Input: part model. Units: mm. Frame: model coordinates. Face numbers are marked on the shaded views. Give positions to 0.01 mm unless a question says otherwise; leave off trailing zeros. Order: outer loops, then holes, each group sorted by start corner. A loop starts at its lowest first (then second) coordinate and runs counter-clockwise, first axis right, second up. Notation, with made-up numbers: M 42.5,-32 L 82.5,-32 A6 cw 82.5,-26 Z; hole C 74.25,-25 d2. An arc over 180 degrees is marked long. Use a Markdown table: item, result.
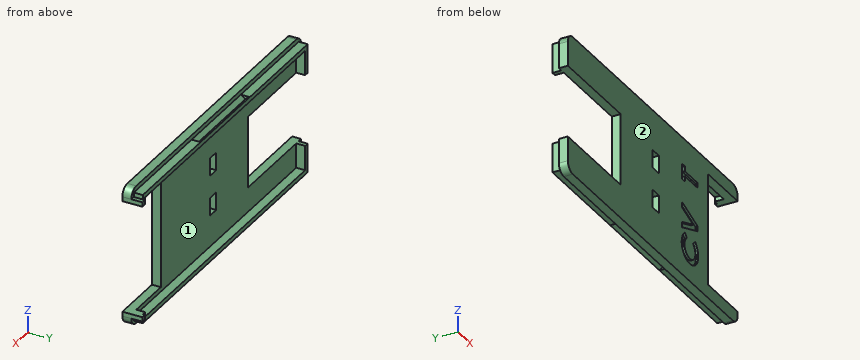
from build123d import *

# Parameters (mm, degrees)
BOSS_EXTRUDE1_DEPTH = 1
SKETCH3_W           = 67
SKETCH3_H           = 29
SKETCH3_W_2         = 65
SKETCH3_H_2         = 27
BOSS_EXTRUDE2_DEPTH = 2
CUT_EXTRUDE1_DEPTH  = 10
SKETCH7_W           = 21.5
SKETCH7_H           = 16
SKETCH7_W_2         = 12
SKETCH7_H_2         = 25
CUT_EXTRUDE2_DEPTH  = 20
SKETCH11_W          = 1
SKETCH11_H          = 1
BOSS_EXTRUDE5_DEPTH = 2.5
CUT_EXTRUDE3_DEPTH  = 0.5
SKETCH13_W          = 2.5
SKETCH13_H          = 4
CUT_EXTRUDE4_DEPTH  = 39.08871237


with BuildPart() as part:
    # Sketch1 → Boss-Extrude1 (new, symmetric)
    with BuildSketch(Plane(origin=(0, 0, 0), x_dir=(1, 0, 0), z_dir=(0, 1, 0))):
        with BuildLine():
            Line((-32.5, -15.5), (32.5, -15.5))
            ThreePointArc((32.5, -15.5), (33.914213562, -14.914213562), (34.5, -13.5))
            Line((34.5, -13.5), (34.5, 13.5))
            ThreePointArc((34.5, 13.5), (33.914213562, 14.914213562), (32.5, 15.5))
            Line((32.5, 15.5), (-32.5, 15.5))
            ThreePointArc((-32.5, 15.5), (-33.914213562, 14.914213562), (-34.5, 13.5))
            Line((-34.5, 13.5), (-34.5, -13.5))
            ThreePointArc((-34.5, -13.5), (-33.914213562, -14.914213562), (-32.5, -15.5))
        make_face()
    extrude(amount=BOSS_EXTRUDE1_DEPTH, both=True)

    # Sketch3 → Boss-Extrude2 (add)
    with BuildSketch(Plane(origin=(0, 1, 0), x_dir=(1, 0, 0), z_dir=(0, 1, 0))):
        Rectangle(SKETCH3_W, SKETCH3_H)
        Rectangle(SKETCH3_W_2, SKETCH3_H_2, mode=Mode.SUBTRACT)
    extrude(amount=BOSS_EXTRUDE2_DEPTH)

    # Sketch6 → Cut-Extrude1 (cut, symmetric)
    with BuildSketch(Plane(origin=(0, 0, 0), x_dir=(0, 0, -1), z_dir=(1, 0, 0))):
        Polygon((14.5, 1), (14.5, 3), (13.75, 2), align=None)
        Polygon((-13.75, 2), (-14.5, 1), (-14.5, 3), align=None)
    extrude(amount=CUT_EXTRUDE1_DEPTH, both=True, mode=Mode.SUBTRACT)

    # Sketch7 → Cut-Extrude2 (cut)
    with BuildSketch(Plane.XZ.offset(1)):
        with Locations((-23.75, 0)):
            Rectangle(SKETCH7_W, SKETCH7_H)
        with Locations((28.5, 0)):
            Rectangle(SKETCH7_W_2, SKETCH7_H_2)
    extrude(amount=-CUT_EXTRUDE2_DEPTH, mode=Mode.SUBTRACT)

    # Sketch11 → Boss-Extrude5 (add)
    with BuildSketch(Plane(origin=(0, 1, 0), x_dir=(1, 0, 0), z_dir=(0, 1, 0))):
        with Locations((34, 13)):
            Rectangle(SKETCH11_W, SKETCH11_H)
        with Locations((34, -13)):
            Rectangle(SKETCH11_W, SKETCH11_H)
    extrude(amount=BOSS_EXTRUDE5_DEPTH)

    # Sketch12 → Cut-Extrude3 (cut)
    with BuildSketch(Plane.XZ.offset(1)):
        Polygon((11.941533437, 6.065064103), (11.941533437, 9.484294872), (13.081277027, 9.484294872), (13.081277027, 8.344551282), (18.291533437, 8.344551282), (18.291533437, 7.204807692), (13.081277027, 7.204807692), (13.081277027, 6.065064103), align=None)
        Polygon((11.941533437, -4.884615385), (11.941533437, -3.667277644), (16.452170457, -2.03525641), (11.941533437, -0.399419071), (11.941533437, 0.814102564), (18.291533437, -1.48828125), (18.291533437, -2.586047676), align=None)
        with BuildLine():
            Line((13.043115969, -5.495192308), (13.84195411, -6.330919471))
            add(Edge.make_bspline(
                [(13.84195411, -6.330919471), (13.768637735, -6.401806055), (13.625427884, -6.540269761), (13.436040425, -6.763499644), (13.277548365, -6.995057512), (13.146745209, -7.232632751), (13.043791904, -7.47669033), (12.970992617, -7.72804876), (12.926114938, -7.986340764), (12.921019422, -8.161199427), (12.918456514, -8.249148638)],
                knots=[0, 0, 0, 0, 1.115315123, 2.178559852, 3.196385012, 4.180486591, 5.141138664, 6.08807191, 7.038351522, 8, 8, 8, 8], degree=3))
            add(Edge.make_bspline(
                [(12.918456514, -8.249148638), (12.920487286, -8.322594137), (12.92449479, -8.467530739), (12.953944547, -8.680315542), (13.00383624, -8.883932376), (13.07318533, -9.078542785), (13.160519089, -9.265108945), (13.270291327, -9.441893594), (13.398838264, -9.609846789), (13.545934957, -9.767006139), (13.707838119, -9.908887036), (13.878351171, -10.03672374), (14.060490077, -10.142609994), (14.251598692, -10.229044823), (14.451746028, -10.297157456), (14.660922066, -10.345499724), (14.879599088, -10.373509267), (15.028259493, -10.377685306), (15.103813085, -10.379807692)],
                knots=[0, 0, 0, 0, 1.035268443, 2.04298821, 3.02163646, 3.985902049, 4.951223231, 5.920091634, 6.913651787, 7.92868536, 8.949353712, 9.945284791, 10.92850487, 11.913014323, 12.897904816, 13.904240668, 14.934873455, 16, 16, 16, 16], degree=3))
            add(Edge.make_bspline(
                [(15.103813085, -10.379807692), (15.156840057, -10.379186533), (15.261357308, -10.377962216), (15.415574733, -10.364925614), (15.565507754, -10.343215337), (15.710796025, -10.312972773), (15.851629254, -10.274204313), (15.988337217, -10.229420059), (16.119289945, -10.172219135), (16.24693936, -10.109298874), (16.368212678, -10.036911087), (16.483189742, -9.95764624), (16.591896287, -9.872234836), (16.693945792, -9.779536195), (16.787869185, -9.678383039), (16.876223869, -9.571218373), (16.957616144, -9.456977598), (17.030749894, -9.335614926), (17.098918302, -9.210802926), (17.155368302, -9.07997032), (17.206114124, -8.94677674), (17.244290102, -8.808884538), (17.277495177, -8.66872294), (17.29777454, -8.524340956), (17.313184177, -8.377108845), (17.31413292, -8.277600269), (17.31461036, -8.227524038)],
                knots=[0, 0, 0, 0, 1.103738238, 2.175490744, 3.219137561, 4.256155604, 5.262629953, 6.259184223, 7.247888397, 8.234817694, 9.220364322, 10.185094651, 11.140491148, 12.096499151, 13.05201798, 14.011605636, 14.986460005, 15.968997565, 16.960259839, 17.944382265, 18.933125845, 19.924977513, 20.920749559, 21.929466621, 22.958034467, 24, 24, 24, 24], degree=3))
            add(Edge.make_bspline(
                [(17.31461036, -8.227524038), (17.312162797, -8.142583361), (17.307353971, -7.975697017), (17.269475061, -7.730825721), (17.207829637, -7.497111584), (17.132929858, -7.311049721), (17.060303901, -7.165191721), (16.995016409, -7.053220916), (16.919750327, -6.938662767), (16.834193119, -6.821691737), (16.738718629, -6.701628906), (16.631461316, -6.58046115), (16.51588805, -6.45512538), (16.43340391, -6.373017633), (16.391112764, -6.330919471)],
                knots=[0, 0, 0, 0, 1.404693586, 2.759857621, 4.088769373, 5.395275838, 6.0697462, 6.783214465, 7.53810233, 8.336454657, 9.18000028, 10.074808326, 11.012918585, 12, 12, 12, 12], degree=3))
            Line((16.391112764, -6.330919471), (17.242104351, -5.520633013))
            add(Edge.make_bspline(
                [(17.242104351, -5.520633013), (17.297096261, -5.577591789), (17.404428711, -5.68876314), (17.556830773, -5.856462037), (17.693780967, -6.023949878), (17.820249986, -6.187180506), (17.93255348, -6.348827808), (18.030803608, -6.508874644), (18.117485256, -6.665509211), (18.191136583, -6.821984078), (18.253674209, -6.979272912), (18.307515, -7.141104638), (18.353062372, -7.307973991), (18.38981312, -7.480900133), (18.419282258, -7.658270114), (18.439173756, -7.841743881), (18.452546148, -8.030158121), (18.453747768, -8.157962419), (18.45435395, -8.222435897)],
                knots=[0, 0, 0, 0, 1.244526981, 2.429050516, 3.560637417, 4.644440555, 5.67424972, 6.652764056, 7.595344123, 8.486817594, 9.369275933, 10.254498637, 11.166417451, 12.086725134, 13.032340136, 13.991389299, 14.986715468, 16, 16, 16, 16], degree=3))
            add(Edge.make_bspline(
                [(18.45435395, -8.222435897), (18.451334939, -8.340865691), (18.445427572, -8.572599876), (18.401657986, -8.912200283), (18.328279045, -9.234811554), (18.224500984, -9.541218541), (18.091929374, -9.831323814), (17.929402805, -10.105053156), (17.737353086, -10.361965375), (17.518031224, -10.599985126), (17.275808639, -10.815285319), (17.015728035, -11.005585757), (16.736511209, -11.163002287), (16.442283088, -11.293708623), (16.131700993, -11.395919259), (15.804428969, -11.467858219), (15.460783018, -11.51222245), (15.226064912, -11.51707596), (15.106357155, -11.519551282)],
                knots=[0, 0, 0, 0, 1.078019885, 2.10938526, 3.111377082, 4.085535484, 5.04941344, 6.010039228, 6.978205633, 7.964457913, 8.951525778, 9.924444315, 10.892603023, 11.863865945, 12.85144698, 13.863884204, 14.910567087, 16, 16, 16, 16], degree=3))
            add(Edge.make_bspline(
                [(15.106357155, -11.519551282), (15.028282903, -11.518515641), (14.873558818, -11.516463254), (14.645252317, -11.494488037), (14.422973185, -11.464639878), (14.208620877, -11.415608228), (13.999755502, -11.358606766), (13.798225395, -11.285168838), (13.603181636, -11.199848512), (13.414870564, -11.102428539), (13.235325687, -10.990848613), (13.063401988, -10.869367728), (12.901326556, -10.735039657), (12.748431173, -10.589223971), (12.602984036, -10.433268126), (12.468562175, -10.264501174), (12.341559366, -10.085801372), (12.225763331, -9.895930835), (12.120448829, -9.699216136), (12.029843958, -9.496613136), (11.952101659, -9.290733703), (11.888096138, -9.080953584), (11.840190071, -8.866901839), (11.803961981, -8.650012752), (11.783702598, -8.428465968), (11.780386745, -8.279715595), (11.778712925, -8.204627404)],
                knots=[0, 0, 0, 0, 1.071814294, 2.12407397, 3.147667899, 4.14936388, 5.141177959, 6.119239245, 7.091825145, 8.063277363, 9.028022524, 9.992609517, 10.952139039, 11.915934802, 12.892469547, 13.878248468, 14.87668965, 15.901326483, 16.93027266, 17.938917451, 18.9468897, 19.950817235, 20.948103127, 21.957084021, 22.968749718, 24, 24, 24, 24], degree=3))
            add(Edge.make_bspline(
                [(11.778712925, -8.204627404), (11.779673395, -8.140569838), (11.781584349, -8.013120728), (11.797486076, -7.823322383), (11.822530484, -7.635062735), (11.860053114, -7.448916668), (11.905494747, -7.264047093), (11.961466571, -7.081228011), (12.029739078, -6.900963551), (12.105262879, -6.721690962), (12.191242805, -6.546985568), (12.287480484, -6.37836568), (12.391458247, -6.215413485), (12.504964528, -6.059111316), (12.626332067, -5.908358268), (12.755556847, -5.763315194), (12.894982972, -5.625373889), (12.993488679, -5.538805542), (13.043115969, -5.495192308)],
                knots=[0, 0, 0, 0, 0.996333415, 1.982307736, 2.96084097, 3.949129141, 4.93457382, 5.921430247, 6.92116383, 7.931890485, 8.946633814, 9.948019707, 10.950686436, 11.952094051, 12.951305284, 13.960287133, 14.972390273, 16, 16, 16, 16], degree=3))
        make_face()
    extrude(amount=-CUT_EXTRUDE3_DEPTH, mode=Mode.SUBTRACT)

    # Sketch13 → Cut-Extrude4 (cut, through all)
    with BuildSketch(Plane.XZ.offset(1)):
        with Locations((1.25, 4.5)):
            Rectangle(SKETCH13_W, SKETCH13_H)
        with Locations((1.25, -4.5)):
            Rectangle(SKETCH13_W, SKETCH13_H)
    extrude(amount=-CUT_EXTRUDE4_DEPTH, mode=Mode.SUBTRACT)


solid = part.part
1) Cut plane B-B on x = 27. Return loops of the section in (y, z), and give its area (3 significant figures).
Response values:
| item | result |
|---|---|
| outline | M -1,-15.5 L 1,-15.5 L 1,-14.5 L 3,-14.5 L 3,-13.5 L 1,-13.5 L 1,-12.5 L -1,-12.5 Z; M -1,12.5 L 1,12.5 L 1,13.5 L 3,13.5 L 3,14.5 L 1,14.5 L 1,15.5 L -1,15.5 Z |
| area | 16.0 mm² |
2) First-contact query: pin 1 Ø1.5 at (x, z) = (-5.5, 6) entering from +Y; pin 2 Ø0.6 at (y, z) = (-1, 7.5) entering from +X; pin 3 Ø10 at (x, z) = (27, 2) entering from -Y; pin 4 Ø0.6 at (y, z) = (3.5, -13) entering from -X. Flat tips, straight axial feed; report the tip coordinate or a pass-through.
Response values:
| item | result |
|---|---|
| pin 1 | stops at y = 1 |
| pin 2 | stops at x = 22.5 |
| pin 3 | stops at y = -1 |
| pin 4 | stops at x = 33.5 |
3) Mould query, pull axis Z, two halves, no side actions, for the marked faces 1 and 2. Classes: released by +Z, released by -Z, zero draft, split by the parting line, or undercut.
Response values:
| item | result |
|---|---|
| face 1 | undercut |
| face 2 | zero draft |
4) Cut plane A-A on x = -26. Return loops of the section in (y, z), and give its area (3 significant figures).
Response values:
| item | result |
|---|---|
| outline | M -1,-15.5 L 1,-15.5 L 1,-14.5 L 3,-14.5 L 3,-13.5 L 1,-13.5 L 1,-8 L -1,-8 Z; M -1,8 L 1,8 L 1,13.5 L 3,13.5 L 3,14.5 L 1,14.5 L 1,15.5 L -1,15.5 Z |
| area | 34.0 mm² |
5) Cut plane D-D on x = -3.5. Return loops of the section in (y, z).
Response values:
| item | result |
|---|---|
| outline | M -1,-15.5 L 1,-15.5 L 1,-14.5 L 2,-13.75 L 3,-14.5 L 3,-13.5 L 1,-13.5 L 1,13.5 L 3,13.5 L 3,14.5 L 2,13.75 L 1,14.5 L 1,15.5 L -1,15.5 Z |
6) Cut plane C-C on x = -11. Return loops of the section in (y, z), and give its area (3 significant figures).
Response values:
| item | result |
|---|---|
| outline | M -1,-15.5 L 1,-15.5 L 1,-14.5 L 3,-14.5 L 3,-13.5 L 1,-13.5 L 1,13.5 L 3,13.5 L 3,14.5 L 1,14.5 L 1,15.5 L -1,15.5 Z |
| area | 66.0 mm² |
7) Material intervals for line 1 (Z direction, x = 32.5, y = 0.65); line 2 (Z direction, x = -22.5, y = 1.5); line 3 (Y direction, x = 3.5, z = 8.5), sorted ascending. Write a range as from..to.
Response values:
| item | result |
|---|---|
| line 1 | z = -15.5..-12.5, 12.5..15.5 |
| line 2 | z = -14.5..-13.5, 13.5..14.5 |
| line 3 | y = -1..1 |
